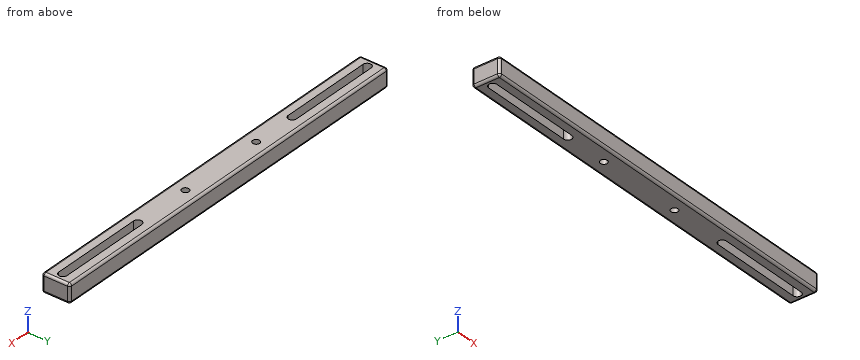
```python
from build123d import *

# Parameters (mm, degrees)
SKETCH_W        = 170
SKETCH_H        = 12
PAD_DEPTH       = 8
POCKET_DEPTH    = 8
POCKET001_DEPTH = 8
FILLET_R        = 1
FILLET001_R     = 1
FILLET002_R     = 1
FILLET003_R     = 1
FILLET004_R     = 1
SKETCH003_R     = 1.5
POCKET002_DEPTH = 8


with BuildPart() as part:
    # Sketch → Pad (new body)
    with BuildSketch(Plane.XY):
        with Locations((85, 6)):
            Rectangle(SKETCH_W, SKETCH_H)
    extrude(amount=PAD_DEPTH)

    # Sketch001 (on Face6 of Pad) → Pocket (cut)
    with BuildSketch(Plane.XY.offset(8)):
        with BuildLine():
            ThreePointArc((3.75, 7.75), (2, 6), (3.75, 4.25))
            Line((3.75, 4.25), (43.75, 4.25))
            ThreePointArc((43.75, 4.25), (45.5, 6), (43.75, 7.75))
            Line((43.75, 7.75), (3.75, 7.75))
        make_face()
    extrude(amount=-POCKET_DEPTH, mode=Mode.SUBTRACT)

    # Sketch002 (on Face5 of Pocket) → Pocket001 (cut)
    with BuildSketch(Plane.XY.offset(8)):
        with BuildLine():
            ThreePointArc((126.25, 7.75), (124.5, 6), (126.25, 4.25))
            Line((126.25, 4.25), (166.25, 4.25))
            ThreePointArc((166.25, 4.25), (168, 6), (166.25, 7.75))
            Line((166.25, 7.75), (126.25, 7.75))
        make_face()
    extrude(amount=-POCKET001_DEPTH, mode=Mode.SUBTRACT)

    # Fillet
    fillet_edges = [part.edges().sort_by_distance(p)[0] for p in [
        (0, 6, 8),
    ]]
    fillet(fillet_edges, radius=FILLET_R)

    # Fillet001
    fillet001_edges = [part.edges().sort_by_distance(p)[0] for p in [
        (0, 0, 3.5),
    ]]
    fillet(fillet001_edges, radius=FILLET001_R)

    # Fillet002
    fillet002_edges = [part.edges().sort_by_distance(p)[0] for p in [
        (0, 6.5, 0),
    ]]
    fillet(fillet002_edges, radius=FILLET002_R)

    # Fillet003
    fillet003_edges = [part.edges().sort_by_distance(p)[0] for p in [
        (0, 12, 4),
    ]]
    fillet(fillet003_edges, radius=FILLET003_R)

    # Fillet004
    fillet004_edges = [part.edges().sort_by_distance(p)[0] for p in [
        (170, 6, 8),
    ]]
    fillet(fillet004_edges, radius=FILLET004_R)

    # Sketch003 (on Face22 of Fillet004) → Pocket002 (cut)
    with BuildSketch(Plane.XY.offset(8)):
        with Locations((63, 6)):
            Circle(SKETCH003_R)
        with Locations((100.8, 6)):
            Circle(SKETCH003_R)
    extrude(amount=-POCKET002_DEPTH, mode=Mode.SUBTRACT)


solid = part.part
```
The listing builds one solid part. Answer for the finished solid, in the listing's coordinates (mm). Coordinates: 2 decimals unless noted, no trailing zeros. Write each loop counter-clockwise with the first axis right and the second up, starting at its lowest first coordinate (ties: lowest second). Pieces come first, ordered by that corner, then holes. Notation, with made-up numbers: (-39, -5.5) -> (-3, -5.5) arc R20 cw to (-3, 1.5) -> close; hole circle Ø2 at (11, -20.75). An arc over 180 degrees is marked (long way). Write each question's results on one line, items separated by ' | '. Start each with the question number.
1) A cutting plane is placed at B-B (x = 146). Determine the outline of the cut face in (y, z).
2) Straight lines are drawn through the part: probe 1 along Y at (x, z) = (135.5, 5.75); probe 2 along X at (y, z) = (5.25, 4.25); probe 3 along Y at (x, z) = (63, 3.25). For each, find the intervals that lie inside material, in ascending order.
3) A cutting plane is placed at A-A (z = 4.25). Determine the outline of the cut face in (x, y), then the cut area to 3 significant figures.
4) A cutting plane is placed at C-C (x = 63). Determine the outline of the cut face in (y, z).
Values follow:
1) outline: (0, 1) arc R1 ccw to (1, 0) -> (4.25, 0) -> (4.25, 8) -> (1, 8) arc R1 ccw to (0, 7) -> close; (7.75, 0) -> (11, 0) arc R1 ccw to (12, 1) -> (12, 7) arc R1 ccw to (11, 8) -> (7.75, 8) -> close
2) probe 1: 0 to 4.25, 7.75 to 12 | probe 2: 0 to 2.17, 45.33 to 61.7, 64.3 to 99.5, 102.1 to 124.67, 167.83 to 170 | probe 3: 0 to 4.5, 7.5 to 12
3) outline: (0, 1) arc R1 ccw to (1, 0) -> (169, 0) arc R1 ccw to (170, 1) -> (170, 11) arc R1 ccw to (169, 12) -> (1, 12) arc R1 ccw to (0, 11) -> close; hole (3.75, 4.25) -> (43.75, 4.25) arc R1.75 ccw to (43.75, 7.75) -> (3.75, 7.75) arc R1.75 ccw to start; hole circle Ø3 at (63, 6); hole circle Ø3 at (100.8, 6); hole (126.25, 4.25) -> (166.25, 4.25) arc R1.75 ccw to (166.25, 7.75) -> (126.25, 7.75) arc R1.75 ccw to start | area: 1,730 mm²
4) outline: (0, 1) arc R1 ccw to (1, 0) -> (4.5, 0) -> (4.5, 8) -> (1, 8) arc R1 ccw to (0, 7) -> close; (7.5, 0) -> (11, 0) arc R1 ccw to (12, 1) -> (12, 7) arc R1 ccw to (11, 8) -> (7.5, 8) -> close
